Autodesk Inventor part; units mm, degrees
ref_plane "Work Plane1" through (0, 0, 0) normal (-1, 0, 0) x (0, 1, 0)
ref_plane "Work Plane2" through (0, 20.3835, 0) normal (0, 1, -0.0003) x (1, 0, 0)
ref_plane "YZ Plane" through (0, 0, 0) normal (1, 0, 0) x (0, 1, 0)
sketch "Sketch1" plane through (0, 0, 0) normal (0, 0, 1) x (1, 0, 0)
  circle A0 centre (0, 0) radius 20.3835
  dimension "d0" = 40.767
extrude "Extrusion1" add sketch "Sketch1" against normal blind 101.6
sketch "Sketch2" plane through (0, 0, 0) normal (0, 0, 1) x (1, 0, 0)
  line L0 (0, 0) -> (0, 19.704)
sketch "Sketch3" plane through (0, 0, -101.6) normal (0, 0, -1) x (-1, 0, 0)
  line L0 (0, 0) -> (0, 20.098)
sketch "Sketch11" plane through (0, 0, 0) normal (0, 0, 1) x (1, 0, 0)
  circle A0 centre (0, 0) radius 20.3835
  line L0 (0, 20.3835) -> (23.5166, 20.3835)
sketch "Sketch12" plane through (0, 0, -101.6) normal (0, 0, -1) x (-1, 0, 0)
  line L0 (0, 20.3509) -> (-24.2704, 20.3509)
  point P0 (0, 0)
ref_plane "Work Plane1" through (0, 0, 0) normal (-1, 0, 0) x (0, 1, 0)
ref_plane "Work Plane2" through (0, 20.3835, 0) normal (0, 1, -0.0003) x (1, 0, 0)
sketch "Sketch4" plane through (0, 0, 0) normal (-1, 0, 0) x (0, 1, 0)
  circle A0 centre (0, 50.8) radius 20.3835
  point P0 (0, 0)
extrude "Extrusion2" add sketch "Sketch4" along normal mid plane 101.6
sketch "Sketch13" plane through (0, 20.3835, 0) normal (0, 1, -0.0003) x (1, 0, 0)
  ellipse E0 centre (0, 50.8065) end of major axis (20.3835, 30.423) minor radius 0.0046 (0, 50.8131) -> (0, 50.8) ccw
  circle A0 centre (0, 50.8) radius 20.3835
  point P0 (0, 0.0065)
  dimension "d23" = 40.767
extrude "Extrusion9" add sketch "Sketch13" along normal blind 30.4165 and the other way blind 20.3835
sketch "Sketch5" plane through (0, 0, 0) normal (0, 0, 1) x (1, 0, 0)
  circle A0 centre (0, 0) radius 16.7767
  dimension "d5" = 33.5534
sketch "Sketch6" plane through (50.8, 0, -50.8) normal (1, 0, 0) x (0, 0, -1)
  circle A0 centre (0, 0) radius 16.7767
  point P0 (-50.8, 0)
  dimension "d6" = 33.5534
sketch "Sketch7" plane through (0, 0, -101.6) normal (0, 0, -1) x (-1, 0, 0)
  circle A0 centre (0, 0) radius 20.3835
  circle A1 centre (0, 0) radius 16.7767
  dimension "d7" = 33.5534
sketch "Sketch8" plane through (-50.8, 0, -50.8) normal (-1, 0, 0) x (0, 0, 1)
  circle A0 centre (0, 0) radius 16.7767
  point P0 (50.8, 0)
  dimension "d8" = 33.5534
extrude "Extrusion3" cut sketch "Sketch5" against normal blind 31.75
extrude "Extrusion4" cut sketch "Sketch6" against normal blind 31.75
extrude "Extrusion5" cut sketch "Sketch7" against normal blind 31.75 contours A1
extrude "Extrusion6" cut sketch "Sketch8" against normal blind 31.75
sketch "Sketch9" plane through (0, 0, 0) normal (0, 0, 1) x (1, 0, 0)
  circle A0 centre (0, 0) radius 12.7
  dimension "d17" = 25.4
sketch "Sketch10" plane through (50.8, 0, -50.8) normal (1, 0, 0) x (0, 0, -1)
  circle A0 centre (0, 0) radius 12.7
  point P0 (-50.8, 0)
  dimension "d18" = 25.4
extrude "Extrusion7" cut sketch "Sketch10" against normal blind 101.6
extrude "Extrusion8" cut sketch "Sketch9" against normal blind 101.6
sketch "Sketch14" plane through (0, 50.7837, -50.8097) normal (0, 1, -0.0003) x (1, 0, 0)
  ellipse E0 centre (0, 0.0065) end of major axis (20.3835, -20.377) minor radius 0.0046 (0, 0.0131) -> (-14.4124, 14.4143) ccw
  circle A0 centre (0, 0.0131) radius 16.7767
  point P0 (0, -50.7935)
  dimension "d28" = 33.5534
extrude "Extrusion10" cut sketch "Sketch14" against normal blind 31.75
sketch "Sketch15" plane through (0, 50.7837, -50.8097) normal (0, 1, -0.0003) x (1, 0, 0)
  ellipse E0 centre (0, 0.0065) end of major axis (-20.3835, -20.377) minor radius 0.0046 (14.4124, 14.4143) -> (0, 0.0131) ccw
  circle A0 centre (0, 0.0131) radius 12.7
  point P0 (0, -50.7935)
  dimension "d31" = 25.4
extrude "Extrusion11" cut sketch "Sketch15" against normal blind 50.8
properties part number "5-way 1 Inch"
Source: CAD feature listing. Evaluate the final solid. Frame: model axes, mm. A direction names the side the tool comes from. Coordinates: 2 decimals unless noted, no trailing zeros. Loops run counter-clockwise (first coordinate to the right, second up) from the corner with the lowest first, then second, coordinate; pieces in that order, holes last. Notation, with made-up numbers: (85.5, 14.25) -> (127.5, 14.25) arc R25 ccw to (127.5, 41.25) -> close; hole circle Ø9 at (3, 65.5). An arc over 180 degrees is marked (long way). One line per item, written item: value. Start each with the question number.
Q1. Section query C-C, the plane x = 45.5. Return the cut outline in (y, z), and give its area (3 significant figures).
Q2. Set-up query: faces 1 (the face through (-3, 13, -31.75)), 2 (the face through (-35.15, 0.74, -67.56)), 3 (the face through (35.15, 5.04, -66.8)), 4 (the face through (-16, 5.04, -85.95)). Return all of +Z, -Z, +X, -X, +Y, -Y with unobstructed straight access to the full face (end or side cutting, diameter ignored); none if empty.
Q3. Section query A-A, the plane x = -6. Give the number of separate pieces and of enclosed holes in the cut face, and give its area (3 significant figures).
Q4. Line query: line 1 along Y through (x, z) = (-42, -50.8); line 2 along Z through (x, y) = (0, 13.75); line 3 along Z through (x, y) = (0, 37). Output: solid intervals per line, ascending.
Q5. Section query D-D, the plane z = -78. Return the cut outline in (x, y).
Q6. Mould query, pull axis Y, two halves, no side actions, for faces 5 (the face through (-2.75, -12.4, -64.42)), 6 (the face through (-17, -3, -101.6)), 7 (the face through (30.689, -20.364, -51.696)). Classes: pulls with the +Y half, pulls with the -Y half, needs draft (parallel to the pull), parting line crosses it, or undercut.
Q7. Contact query for flat-ended pins moving along their axis: P1, Ø12, axis at x = 31.5, z = -57.5, coming from the -Y side; P2, Ø1, axis at x = 37, y = 0.5, coming from the +Z side; P3, Ø1, axis at x = -5.5, z = -67.5, coming from the -Y side; P4, Ø5, axis at y = 39, z = -25.5, coming from the +X side. Output: stop coordinate, or through.
Results:
1. outline: circle Ø40.77 at (0, -50.8); hole circle Ø33.55 at (0, -50.8)
1. area: 421 mm^2
2. face 1: +Z
2. face 2: -X
2. face 3: +X
2. face 4: -Z
3. separate pieces: 3
3. enclosed holes: 0
3. area: 1,160 mm^2
4. line 1: -20.38 to -16.78, 16.78 to 20.38
4. line 2: -69.85 to -63.51, -38.11 to -31.75
4. line 3: -71.19 to -67.6, -34.04 to -30.42
5. outline: circle Ø40.77 at (0, 0); hole circle Ø33.55 at (0, 0)
6. face 5: undercut
6. face 6: needs draft
6. face 7: parting line crosses it
7. P1: y = -20.37
7. P2: z = -30.42
7. P3: y = -19.76
7. P4: through
